Autodesk Fusion 360 part; units mm, degrees
sketch "Sketch1" plane through (0, 0, 0) normal (1, 0, 0) x (0, 1, 0)
  line L0 (-35, 35) -> (35, 35)
  line L1 (35, 35) -> (35, -35)
  line L2 (35, -35) -> (-35, -35)
  line L3 (-35, -35) -> (-35, 35)
  line L4 (-35, 35) -> (35, -35) construction
  line L5 (35, 35) -> (-35, -35) construction
  dimension "d1" = 70
  dimension "d2" = 70
extrude "Extrude1" add sketch "Sketch1" along normal blind 40
sketch "Sketch2" plane through (40, 0, 0) normal (1, 0, 0) x (0, 1, 0)
  line L0 (-35, -35) -> (35, -35)
  line L1 (35, -35) -> (35, 35)
  line L2 (35, 35) -> (-35, 35)
  line L3 (-35, 35) -> (-35, -35)
  line L4 (-30, 30) -> (30, 30)
  line L5 (30, 30) -> (30, -30)
  line L6 (30, -30) -> (-30, -30)
  line L7 (-30, -30) -> (-30, 30)
  line L8 (-30, 30) -> (30, -30) construction
  line L9 (30, 30) -> (-30, -30) construction
  dimension "d5" = 5
  dimension "d6" = 5
extrude "Extrude2" cut sketch "Sketch2" against normal blind 35 contours L4 L5 L6 L7
Input: part model. Units: mm. Frame: model coordinates. A direction names the side the tool comes from. Coordinates: 2 decimals unless noted, no trailing zeros. Write each loop counter-clockwise with the first axis right and the second up, starting at its lowest first coordinate (ties: lowest second). Pieces come first, ordered by that corner, then holes.
1) Set-up query: faces 1 (the flat face through (20, 0, 35)), 2 (the flat face through (23, 30, 0)). Return all of +Z, -Z, +X, -X, +Y, -Y with unobstructed straight access to the full face (end or side cutting, diameter ignored); none if empty.
2) Section B-B on z = -25.5. Output: boundary loops of the cut face in (x, y).
3) Section A-A on x = 13. Output: boundary loops of the cut face in (y, z).
4) Pin query (flat end, axial travel): pin 1 Ø18 at (y, z) = (-7, 3) entering from +X. Return the tip coordinate at first contact, or that it passes through.
5) Material intervals for line 1 along Y through (x, z) = (28.5, 28.5); line 2 along X through (y, z) = (6.5, 14), sorted ascending.
6) Mould query, pull axis X, two halves, no side actions, for faces 3 (the flat face through (23, 0, -30)), 4 (the flat face through (40, -32, 0)), 5 (the flat face through (0, 0, 0)). Classes: pulls with the +X half, pulls with the -X half, needs draft (parallel to the pull), parting line crosses it, or undercut.
Check result:
1. face 1: +Z, +X, -X, +Y, -Y
1. face 2: +X
2. outline: (0, -35) - (40, -35) - (40, -30) - (5, -30) - (5, 30) - (40, 30) - (40, 35) - (0, 35) - close
3. outline: (-35, -35) - (35, -35) - (35, 35) - (-35, 35) - close; hole (-30, -30) - (30, -30) - (30, 30) - (-30, 30) - close
4. pin 1: stops at x = 5
5. line 1: y = -35 to -30, 30 to 35
5. line 2: x = 0 to 5
6. face 3: needs draft
6. face 4: pulls with the +X half
6. face 5: pulls with the -X half
